Geometry check sheet. Reference: the model listing, model coordinates, mm. Give positions to 0.01 mm unless a question says otherwise; leave off trailing zeros. Loops run counter-clockwise (first coordinate to the right, second up) from the corner with the lowest first, then second, coordinate; pieces in that order, holes last. Notation, with made-up numbers: (32.5, 15.25) -> (61.5, 15.25) arc R25 cw to (61.5, 37.25) -> close; hole circle Ø9 at (47.5, 79). An arc over 180 degrees is marked (long way). Answer in a Markdown table with one row per item. Add a question column.
```python
from build123d import *

# Parameters (mm, degrees)
SKETCH1_R           = 2.54
SKETCH1_W           = 50.8
SKETCH1_H           = 355.6
BOSS_EXTRUDE1_DEPTH = 3.175
FILLET1_R           = 6.35
SKETCH3_R           = 1.4224
CUT_EXTRUDE3_DEPTH  = 700.116959077
SKETCH5_R           = 2.54
CUT_EXTRUDE5_DEPTH  = 700.116959077


with BuildPart() as part:
    # Sketch1 → Boss-Extrude1 (new body)
    # profile 1 of 2: a face of its own
    with BuildSketch(Plane.XY):
        Polygon((0, 190.5), (0, 63.5), (63.5, 63.5), (63.5, 0), (445.262, 0), (445.262, 63.5), (508.762, 63.5), (508.762, 419.1), (280.162, 419.1), align=None)
        with Locations((12.7, 144.4625)):
            Circle(SKETCH1_R, mode=Mode.SUBTRACT)
        with Locations((38.1, 144.4625)):
            Circle(SKETCH1_R, mode=Mode.SUBTRACT)
        with Locations((12.7, 169.8625)):
            Circle(SKETCH1_R, mode=Mode.SUBTRACT)
        with Locations((38.1, 169.8625)):
            Circle(SKETCH1_R, mode=Mode.SUBTRACT)
        with Locations((292.862, 12.7)):
            Circle(SKETCH1_R, mode=Mode.SUBTRACT)
        with Locations((318.262, 12.7)):
            Circle(SKETCH1_R, mode=Mode.SUBTRACT)
        with Locations((292.862, 139.7)):
            Circle(SKETCH1_R, mode=Mode.SUBTRACT)
        with Locations((318.262, 139.7)):
            Circle(SKETCH1_R, mode=Mode.SUBTRACT)
        with Locations((292.862, 266.7)):
            Circle(SKETCH1_R, mode=Mode.SUBTRACT)
        with Locations((318.262, 266.7)):
            Circle(SKETCH1_R, mode=Mode.SUBTRACT)
        with Locations((292.862, 393.7)):
            Circle(SKETCH1_R, mode=Mode.SUBTRACT)
        with Locations((318.262, 393.7)):
            Circle(SKETCH1_R, mode=Mode.SUBTRACT)
    # profile 2 of 2: a face of its own
    with BuildSketch(Plane.XY):
        with Locations((534.162, 241.3)):
            Rectangle(SKETCH1_W, SKETCH1_H)
        with Locations((521.462, 342.9)):
            Circle(SKETCH1_R, mode=Mode.SUBTRACT)
        with Locations((546.862, 342.9)):
            Circle(SKETCH1_R, mode=Mode.SUBTRACT)
        with Locations((521.462, 368.3)):
            Circle(SKETCH1_R, mode=Mode.SUBTRACT)
        with Locations((546.862, 368.3)):
            Circle(SKETCH1_R, mode=Mode.SUBTRACT)
    extrude(amount=BOSS_EXTRUDE1_DEPTH)

    # Fillet1
    fillet1_edges = [part.edges().sort_by_distance(p)[0] for p in [
        (280.162, 419.1, 1.5875),
        (559.562, 419.1, 1.5875),
        (559.562, 63.5, 1.5875),
        (445.262, 63.5, 1.5875),
        (445.262, 0, 1.5875),
        (63.5, 0, 1.5875),
        (63.5, 63.5, 1.5875),
        (0, 63.5, 1.5875),
        (0, 190.5, 1.5875),
    ]]
    fillet(fillet1_edges, radius=FILLET1_R)

    # Sketch3 → Cut-Extrude3 (cut, through all)
    with BuildSketch(Plane.XY.offset(3.175)):
        with Locations((521.462, 228.6)):
            Circle(SKETCH3_R)
        with Locations((419.862, 228.6)):
            Circle(SKETCH3_R)
        with Locations((419.862, 101.6)):
            Circle(SKETCH3_R)
        with Locations((521.462, 101.6)):
            Circle(SKETCH3_R)
    extrude(amount=-CUT_EXTRUDE3_DEPTH, mode=Mode.SUBTRACT)

    # Sketch5 → Cut-Extrude5 (cut, through all)
    with BuildSketch(Plane.XY.offset(3.175)):
        with Locations((520.7, 398.145)):
            Circle(SKETCH5_R)
        with Locations((497.84, 398.145)):
            Circle(SKETCH5_R)
    extrude(amount=-CUT_EXTRUDE5_DEPTH, mode=Mode.SUBTRACT)


solid = part.part
```
1. Sectioned sample at C-C (y = 328). Enter the section's corners in (x, z) (3 decimals).
2. Material ranges on L1, parallel to X at y = 101.6, z = 1.7; L2, parallel to X at y = 342.9, z = 1.3; L3, parallel to Y at x = 529.5, z = 2.2, recorded low to high. Write a range as from..to.
3. Sectioned sample at A-A (x = 469.5). Enter the section's corners in (y, z) (3 decimals).
4. Gauge pin test, flat ends, axial feed: pin 1 Ø1.5 at (y, z) = (281, 1.5) entering from -X; pin 2 Ø1 at (x, z) = (525.5, 1) entering from -Y; pin 3 Ø1.6 at (y, z) = (37.5, 2.5) entering from -X. Record the tip position at first contact, or that the pin passes through.
5. Sectioned sample at B-B (z = 1.55). Count the separate pieces of the cut face and the enclosed holes in it, plus the area to 3 significant figures.
Response:
| question | item | result |
|---|---|---|
| 1 | outline | (168.514, 0) -> (559.562, 0) -> (559.562, 3.175) -> (168.514, 3.175) -> close |
| 2 | L1 | x = 0..418.44, 421.28..520.04, 522.88..559.56 |
| 2 | L2 | x = 186.77..518.92, 524..544.32, 549.4..559.56 |
| 2 | L3 | y = 63.5..419.1 |
| 3 | outline | (63.5, 0) -> (419.1, 0) -> (419.1, 3.175) -> (63.5, 3.175) -> close |
| 4 | pin 1 | stops at x = 109.99 |
| 4 | pin 2 | stops at y = 63.5 |
| 4 | pin 3 | stops at x = 63.5 |
| 5 | separate pieces | 1 |
| 5 | enclosed holes | 22 |
| 5 | area | 191,000 mm2 |
